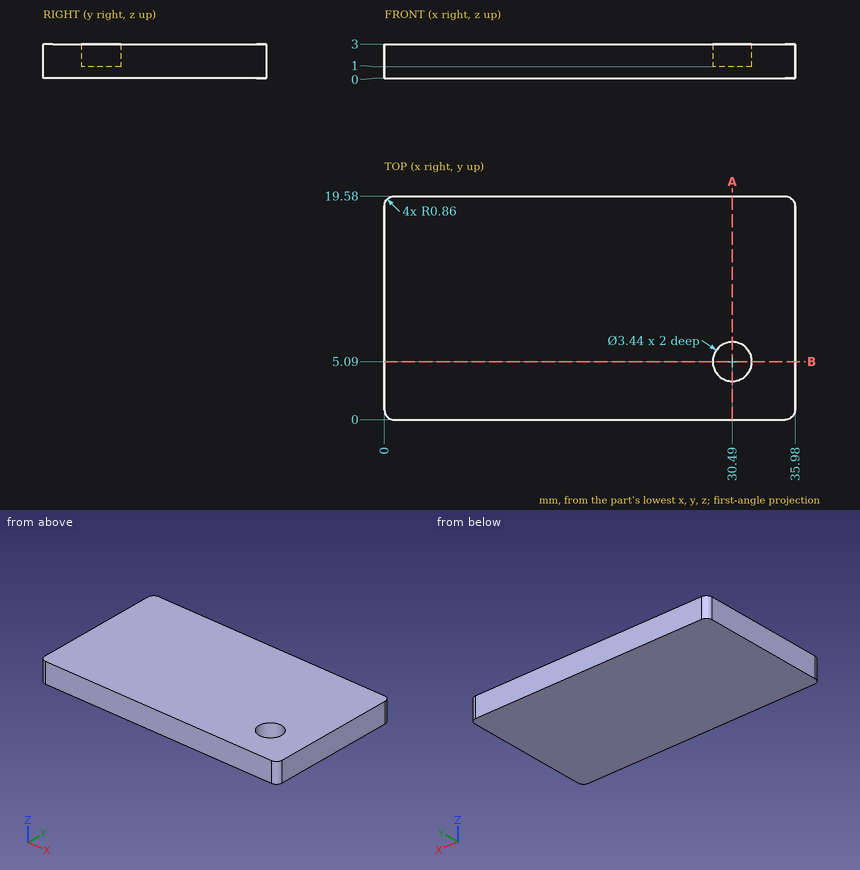
Study the drawing (mm; zero at the part's minimum x, y, z) and answer. Round coordinates to 2 decimals unless told otherwise and drop trailing zeros. Loops run counter-clockwise (first coordinate to the right, second up) from the corner with the lowest first, then second, coordinate; pieces in that order, holes last.
Q1. Section B-B, the plane y = 5.09 is taken. Determine the outline of the cut face in (x, z).
Q2. Section A-A, the plane x = 30.49 is taken. Determine the outline of the cut face in (y, z), then the cut area to 3 significant figures.
Q3. Find the intervals of material crossed by line 1 (Y direction, x = 30.49, z = 2); line 2 (X direction, y = 4.5, z = 1.55); line 3 (Y direction, x = 29.5, z = 1.65), in increasing order.
Q4. Given pin 1 Ø1.7 at (x, y) = (30, 5.5) entering from +Z, flat-ended and moving along its own axis, determine where the tip first touches the part or whether it passes through.
Completed:
1. outline: (0, 0) - (35.98, 0) - (35.98, 3) - (32.21, 3) - (32.21, 1) - (28.77, 1) - (28.77, 3) - (0, 3) - close
2. outline: (0, 0) - (19.58, 0) - (19.58, 3) - (6.81, 3) - (6.81, 1) - (3.37, 1) - (3.37, 3) - (0, 3) - close
2. area: 51.9 mm2
3. line 1: y = 0 to 3.37, 6.81 to 19.58
3. line 2: x = 0 to 28.87, 32.11 to 35.98
3. line 3: y = 0 to 3.68, 6.5 to 19.58
4. pin 1: stops at z = 1
